Build history of the part. All positions in model axes, mm. A direction names the side the tool comes from. Give positions to 0.01 mm unless a question says otherwise; leave off trailing zeros. Order: outer loops, then holes, each group sorted by start corner. A loop starts at its lowest first (then second) coordinate and runs counter-clockwise, first axis right, second up. Notation, with made-up numbers: (19, 43) - (35, 43) arc R17 ccw to (35, 69) - close; hole circle Ø9 at (3.5, 46.5). An arc over 180 degrees is marked (long way). One line per item, written item: value.
```python
from build123d import *

# Parameters (mm, degrees)
SM_BASE_FLANGE_1_DEPTH = 25
CUT_EXTRUDE_2_REACH    = 47.389
SKETCH_7_W             = 2
SKETCH_7_H             = 7.5
CUT_EXTRUDE_3_REACH    = 53.538
SKETCH_8_R             = 1.25
FILLET_1_R             = 2
CUT_EXTRUDE_4_DEPTH    = 10


# Sheet-metal steps are written as plain solids
with BuildPart() as part:
    # Sketch 1 → 基体-法兰1 (new body)
    with BuildSketch(Plane(origin=(0, 0, 0), x_dir=(1, 0, 0), z_dir=(0, 1, 0))):
        with BuildLine():
            Line((-23.132778959, 20.763530703), (-23.132778959, -7.236469297))
            ThreePointArc((-23.132778959, -7.236469297), (-22.546992522, -8.650682859), (-21.132778959, -9.236469297))
            Line((-21.132778959, -9.236469297), (14.867221041, -9.236469297))
            ThreePointArc((14.867221041, -9.236469297), (16.281434603, -8.650682859), (16.867221041, -7.236469297))
            Line((16.867221041, -7.236469297), (16.867221041, 20.763530703))
            Line((16.867221041, 20.763530703), (15.867221041, 20.763530703))
            Line((15.867221041, 20.763530703), (15.867221041, -7.236469297))
            ThreePointArc((15.867221041, -7.236469297), (15.574327822, -7.943576078), (14.867221041, -8.236469297))
            Line((14.867221041, -8.236469297), (-21.132778959, -8.236469297))
            ThreePointArc((-21.132778959, -8.236469297), (-21.839885741, -7.943576078), (-22.132778959, -7.236469297))
            Line((-22.132778959, -7.236469297), (-22.132778959, 20.763530703))
            Line((-22.132778959, 20.763530703), (-23.132778959, 20.763530703))
        make_face()
    extrude(amount=SM_BASE_FLANGE_1_DEPTH)

    # 切除-拉伸2: up to this face of the body (flat: up to its plane)
    cut_extrude_2_end = Plane(part.part.faces().sort_by_distance((-22.632778959, 12.5, -20.763530703))[0])
    # 草图7 → 切除-拉伸2 (cut, up to the picked face)
    with BuildSketch(Plane.XY.offset(9.236469297), mode=Mode.PRIVATE) as cut_extrude_2_sk1:
        with BuildLine():
            Line((-21.132778959, 25), (-21.132778959, 17.5))
            Line((-21.132778959, 17.5), (-14.589218197, 17.5))
            ThreePointArc((-14.589218197, 17.5), (-9.979310906, 22.958250346), (-3.132778905, 25))
            Line((-3.132778905, 25), (-21.132778959, 25))
        make_face()
    cut_extrude_2_tool1 = split(extrude(cut_extrude_2_sk1.sketch, amount=-CUT_EXTRUDE_2_REACH, mode=Mode.PRIVATE), bisect_by=cut_extrude_2_end, keep=Keep.BOTH, mode=Mode.PRIVATE)
    # 草图7 → 切除-拉伸2 (cut, up to the picked face)
    with BuildSketch(Plane.XY.offset(9.236469297), mode=Mode.PRIVATE) as cut_extrude_2_sk2:
        with Locations((-22.132778959, 21.25)):
            Rectangle(SKETCH_7_W, SKETCH_7_H)
    cut_extrude_2_tool2 = split(extrude(cut_extrude_2_sk2.sketch, amount=-CUT_EXTRUDE_2_REACH, mode=Mode.PRIVATE), bisect_by=cut_extrude_2_end, keep=Keep.BOTH, mode=Mode.PRIVATE)
    # 草图7 → 切除-拉伸2 (cut, up to the picked face)
    with BuildSketch(Plane.XY.offset(9.236469297), mode=Mode.PRIVATE) as cut_extrude_2_sk3:
        with BuildLine():
            Line((14.867221041, 25), (-3.132778905, 25))
            ThreePointArc((-3.132778905, 25), (3.713753032, 22.958250317), (8.323660278, 17.5))
            Line((8.323660278, 17.5), (14.867221041, 17.5))
            Line((14.867221041, 17.5), (14.867221041, 25))
        make_face()
    cut_extrude_2_tool3 = split(extrude(cut_extrude_2_sk3.sketch, amount=-CUT_EXTRUDE_2_REACH, mode=Mode.PRIVATE), bisect_by=cut_extrude_2_end, keep=Keep.BOTH, mode=Mode.PRIVATE)
    # 草图7 → 切除-拉伸2 (cut, up to the picked face)
    with BuildSketch(Plane.XY.offset(9.236469297), mode=Mode.PRIVATE) as cut_extrude_2_sk4:
        with Locations((15.867221041, 21.25)):
            Rectangle(SKETCH_7_W, SKETCH_7_H)
    cut_extrude_2_tool4 = split(extrude(cut_extrude_2_sk4.sketch, amount=-CUT_EXTRUDE_2_REACH, mode=Mode.PRIVATE), bisect_by=cut_extrude_2_end, keep=Keep.BOTH, mode=Mode.PRIVATE)
    # 草图7 → 切除-拉伸2 (cut, up to the picked face)
    with BuildSketch(Plane.XY.offset(9.236469297), mode=Mode.PRIVATE) as cut_extrude_2_sk5:
        with Locations((15.867221041, 3.75)):
            Rectangle(SKETCH_7_W, SKETCH_7_H)
    cut_extrude_2_tool5 = split(extrude(cut_extrude_2_sk5.sketch, amount=-CUT_EXTRUDE_2_REACH, mode=Mode.PRIVATE), bisect_by=cut_extrude_2_end, keep=Keep.BOTH, mode=Mode.PRIVATE)
    # 草图7 → 切除-拉伸2 (cut, up to the picked face)
    with BuildSketch(Plane.XY.offset(9.236469297), mode=Mode.PRIVATE) as cut_extrude_2_sk6:
        with BuildLine():
            ThreePointArc((8.323660278, 7.5), (3.713752992, 2.041749657), (-3.132779, 0))
            Line((-3.132779, 0), (14.867221041, 0))
            Line((14.867221041, 0), (14.867221041, 7.5))
            Line((14.867221041, 7.5), (8.323660278, 7.5))
        make_face()
    cut_extrude_2_tool6 = split(extrude(cut_extrude_2_sk6.sketch, amount=-CUT_EXTRUDE_2_REACH, mode=Mode.PRIVATE), bisect_by=cut_extrude_2_end, keep=Keep.BOTH, mode=Mode.PRIVATE)
    # 草图7 → 切除-拉伸2 (cut, up to the picked face)
    with BuildSketch(Plane.XY.offset(9.236469297), mode=Mode.PRIVATE) as cut_extrude_2_sk7:
        with BuildLine():
            Line((-14.589218197, 7.5), (-21.132778959, 7.5))
            Line((-21.132778959, 7.5), (-21.132778959, 0))
            Line((-21.132778959, 0), (-3.132779, 0))
            ThreePointArc((-3.132779, 0), (-9.979310945, 2.041749679), (-14.589218197, 7.5))
        make_face()
    cut_extrude_2_tool7 = split(extrude(cut_extrude_2_sk7.sketch, amount=-CUT_EXTRUDE_2_REACH, mode=Mode.PRIVATE), bisect_by=cut_extrude_2_end, keep=Keep.BOTH, mode=Mode.PRIVATE)
    # 草图7 → 切除-拉伸2 (cut, up to the picked face)
    with BuildSketch(Plane.XY.offset(9.236469297), mode=Mode.PRIVATE) as cut_extrude_2_sk8:
        with Locations((-22.132778959, 3.75)):
            Rectangle(SKETCH_7_W, SKETCH_7_H)
    cut_extrude_2_tool8 = split(extrude(cut_extrude_2_sk8.sketch, amount=-CUT_EXTRUDE_2_REACH, mode=Mode.PRIVATE), bisect_by=cut_extrude_2_end, keep=Keep.BOTH, mode=Mode.PRIVATE)
    add(cut_extrude_2_tool1.solids().sort_by(Axis((-15.911203, 21.806262, 9.236469), (0, 0, -1)))[0], mode=Mode.SUBTRACT)
    add(cut_extrude_2_tool2.solids().sort_by(Axis((-22.132779, 21.25, 9.236469), (0, 0, -1)))[0], mode=Mode.SUBTRACT)
    add(cut_extrude_2_tool3.solids().sort_by(Axis((9.645646, 21.806262, 9.236469), (0, 0, -1)))[0], mode=Mode.SUBTRACT)
    add(cut_extrude_2_tool4.solids().sort_by(Axis((15.867221, 21.25, 9.236469), (0, 0, -1)))[0], mode=Mode.SUBTRACT)
    add(cut_extrude_2_tool5.solids().sort_by(Axis((15.867221, 3.75, 9.236469), (0, 0, -1)))[0], mode=Mode.SUBTRACT)
    add(cut_extrude_2_tool6.solids().sort_by(Axis((9.645646, 3.193738, 9.236469), (0, 0, -1)))[0], mode=Mode.SUBTRACT)
    add(cut_extrude_2_tool7.solids().sort_by(Axis((-15.911203, 3.193738, 9.236469), (0, 0, -1)))[0], mode=Mode.SUBTRACT)
    add(cut_extrude_2_tool8.solids().sort_by(Axis((-22.132779, 3.75, 9.236469), (0, 0, -1)))[0], mode=Mode.SUBTRACT)

    # 切除-拉伸3: up to this face of the body (flat: up to its plane)
    cut_extrude_3_end = Plane(part.part.faces().sort_by_distance((-23.132778959, 12.5, -6.763530703))[0])
    # 草图8 → 切除-拉伸3 (cut, up to the picked face)
    with BuildSketch(Plane(origin=(16.867221041, 0, 0), x_dir=(0, 0, -1), z_dir=(1, 0, 0)), mode=Mode.PRIVATE) as cut_extrude_3_sk1:
        Polygon((20.763530703, 17.5), (-7.236469297, 17.5), (20.763530703, 13.95), align=None)
    cut_extrude_3_tool1 = split(extrude(cut_extrude_3_sk1.sketch, amount=-CUT_EXTRUDE_3_REACH, mode=Mode.PRIVATE), bisect_by=cut_extrude_3_end, keep=Keep.BOTH, mode=Mode.PRIVATE)
    # 草图8 → 切除-拉伸3 (cut, up to the picked face)
    with BuildSketch(Plane(origin=(16.867221041, 0, 0), x_dir=(0, 0, -1), z_dir=(1, 0, 0)), mode=Mode.PRIVATE) as cut_extrude_3_sk2:
        Polygon((20.763530703, 11.051298474), (-7.236469297, 7.5), (20.763530703, 7.5), align=None)
    cut_extrude_3_tool2 = split(extrude(cut_extrude_3_sk2.sketch, amount=-CUT_EXTRUDE_3_REACH, mode=Mode.PRIVATE), bisect_by=cut_extrude_3_end, keep=Keep.BOTH, mode=Mode.PRIVATE)
    # 草图8 → 切除-拉伸3 (cut, up to the picked face)
    with BuildSketch(Plane(origin=(16.867221041, 0, 0), x_dir=(0, 0, -1), z_dir=(1, 0, 0)), mode=Mode.PRIVATE) as cut_extrude_3_sk3:
        with Locations(Location((17.763530703, 12.5, 0), (0, 0, 180))):
            Circle(SKETCH_8_R)
    cut_extrude_3_tool3 = split(extrude(cut_extrude_3_sk3.sketch, amount=-CUT_EXTRUDE_3_REACH, mode=Mode.PRIVATE), bisect_by=cut_extrude_3_end, keep=Keep.BOTH, mode=Mode.PRIVATE)
    add(cut_extrude_3_tool1.solids().sort_by(Axis((16.867221, 16.316667, -11.430197), (-1, 0, 0)))[0], mode=Mode.SUBTRACT)
    add(cut_extrude_3_tool2.solids().sort_by(Axis((16.867221, 8.683766, -11.430197), (-1, 0, 0)))[0], mode=Mode.SUBTRACT)
    add(cut_extrude_3_tool3.solids().sort_by(Axis((16.867221, 12.5, -17.763531), (-1, 0, 0)))[0], mode=Mode.SUBTRACT)

    # 圆角1
    # the kernel refuses this fillet: 2 mm, written as the material it takes off along each edge
    with BuildSketch(Plane(origin=(-17.726883899, 11.051298474, -20.763530703), x_dir=(0, -0.12582409885038226, 0.9920525672304312), z_dir=(-1, 0, 0)), Plane(origin=(21.273116101, 11.051298474, -20.763530703), x_dir=(0, -0.12582409885038226, 0.9920525672304312), z_dir=(-1, 0, 0))) as fillet_1_piece_1:
        with BuildLine():
            CenterArc((FILLET_1_R * 0.881179012106, FILLET_1_R), FILLET_1_R, 187.228348929, 82.771651071)
            Line((-FILLET_1_R * 0.110873555124, FILLET_1_R * 0.87417590115), (0, 0))
            Line((0, 0), (FILLET_1_R * 0.881179012106, 0))
        make_face()
    extrude(amount=9.811790121, mode=Mode.SUBTRACT)
    with BuildSketch(Plane(origin=(-17.726681198, 13.95, -20.763530703), x_dir=(0, -1, 0), z_dir=(-1, 0, 0))) as fillet_1_piece_2:
        with BuildLine():
            CenterArc((FILLET_1_R * 0.881219552242, FILLET_1_R), FILLET_1_R, 187.225733942, 82.774266058)
            Line((-FILLET_1_R * 0.110838756585, FILLET_1_R * 0.874221178702), (0, 0))
            Line((0, 0), (FILLET_1_R * 0.881219552242, 0))
        make_face()
    extrude(amount=9.812195522, mode=Mode.SUBTRACT)
    with BuildSketch(Plane(origin=(21.273318802, 13.95, -20.763530703), x_dir=(0, 0.12577882129772675, 0.9920583088271347), z_dir=(-1, 0, 0))) as fillet_1_piece_3:
        with BuildLine():
            CenterArc((FILLET_1_R * 0.881219552242, -FILLET_1_R), FILLET_1_R, 90, 82.774266058)
            Line((-FILLET_1_R * 0.110838756585, -FILLET_1_R * 0.874221178702), (0, 0))
            Line((0, 0), (FILLET_1_R * 0.881219552242, 0))
        make_face()
    extrude(amount=9.812195522, mode=Mode.SUBTRACT)

    # 草图9 → 切除-拉伸4 (cut)
    with BuildSketch(Plane.XY.offset(9.236469297)):
        with BuildLine():
            ThreePointArc((2.849937878, 14.308203319), (-3.132778959, 18.75), (-9.115495797, 14.308203319))
            Line((-9.115495797, 14.308203319), (-11.508582532, 15.031484647))
            ThreePointArc((-11.508582532, 15.031484647), (-3.132778959, 21.25), (5.243024613, 15.031484647))
            Line((5.243024613, 15.031484647), (2.849937878, 14.308203319))
        make_face()
        with BuildLine():
            Line((-9.115495797, 10.691796681), (-11.508582532, 9.968515353))
            ThreePointArc((-11.508582532, 9.968515353), (-3.132778959, 3.75), (5.243024613, 9.968515353))
            Line((5.243024613, 9.968515353), (2.849937878, 10.691796681))
            ThreePointArc((2.849937878, 10.691796681), (-3.132778959, 6.25), (-9.115495797, 10.691796681))
        make_face()
    extrude(amount=-CUT_EXTRUDE_4_DEPTH, mode=Mode.SUBTRACT)


solid = part.part
```
(1) 3-axis set-ups, long thin cutter, end or side, ignore diameter. For faces 1 (the face through (-18.9, 17.5, 8.5)), 2 (the face through (12.7, 7.5, 8.5)), 3 (the face through (-10.295, 10.335, 8.743)), 4 (the face through (-3, 12, 8.236)): which of +Z, -Z, +X, -X, +Y, -Y reach the whole face in a straight line?
Completed:
face 1: +Z, -Z, -X, +Y
face 2: +Z, -Z, +X, -Y
face 3: +Z, -Z
face 4: -Z, +Y, -Y
(2) Slice it at B-B, the plane y = 19.75. Give the cut face in (x, z), and give its area (3 significant figures).
Completed:
outline: (-13.32, 8.24) - (-8.03, 8.24) - (-8.03, 9.24) - (-13.32, 9.24) - close; (1.77, 8.24) - (7.05, 8.24) - (7.05, 9.24) - (1.77, 9.24) - close
area: 10.6 mm²
(3) Slice it at C-C, the plane x = -10. Give the cut face in (y, z).
Completed:
outline: (2.06, 8.24) - (7.08, 8.24) - (7.08, 9.24) - (2.06, 9.24) - close; (10.42, 8.24) - (14.58, 8.24) - (14.58, 9.24) - (10.42, 9.24) - close; (17.92, 8.24) - (22.94, 8.24) - (22.94, 9.24) - (17.92, 9.24) - close
(4) Pull direction X, two halves, no side cores. Call faces 5 (the face through (-3.02, 18.75, 8.74)), 6 (the face through (16.867, 12, -3)), 7 (the face through (16.37, 13.64, -20.14)): +X half, -X half, draft (parallel to the pull), parting line (faces both ways), or undercut.
Completed:
face 5: undercut
face 6: +X half
face 7: draft
(5) Drill centre lines: line 1 (X direction, y = 15.5, z = -6); line 2 (Z direction, x = 6, y = 10.5); line 3 (Z direction, x = -22.4, y = 12.5). Where is each one in solid material? Low to high.
Completed:
line 1: -23.13 to -22.13, 15.87 to 16.87
line 2: 8.24 to 9.24
line 3: -20.74 to -19.01, -16.51 to 8.78
(6) Pin check, flat tips, straight feed: P1, Ø12.5, axis at x = 0.5, y = 8.5, coming from the -Z side; P2, Ø1, axis at x = 13, z = 8.5, coming from the -Y side; P3, Ø12, axis at y = 15.5, z = -14, coming from the -X side; P4, Ø1.6, axis at x = -19, z = 8.5, coming from the +Y side. Stop position of each tip, or through.
Completed:
P1: z = 8.24
P2: y = 7.5
P3: x = -23.13
P4: y = 17.5
(7) Slice it at A-A, the plane z = -8.75. Give the cut face in (x, y), and give its area (3 significant figures).
Completed:
outline: (-23.13, 9.53) - (-22.13, 9.53) - (-22.13, 15.47) - (-23.13, 15.47) - close; (15.87, 9.53) - (16.87, 9.53) - (16.87, 15.47) - (15.87, 15.47) - close
area: 11.9 mm²
(8) Slice it at D-D, the plane x = -16. Give the cut face in (y, z).
Completed:
outline: (7.5, 8.24) - (17.5, 8.24) - (17.5, 9.24) - (7.5, 9.24) - close
